Input: part model. Units: mm. Frame: model coordinates. Face numbers are marked on the shaded views. A direction names the side the tool comes from. Give positions to 0.01 mm unless a question says otherwise; leave off trailing zeros. Order: outer loops, then holes, each group sorted by start corner. A loop starts at its lowest first (then second) coordinate and runs counter-clockwise, first axis right, second up.
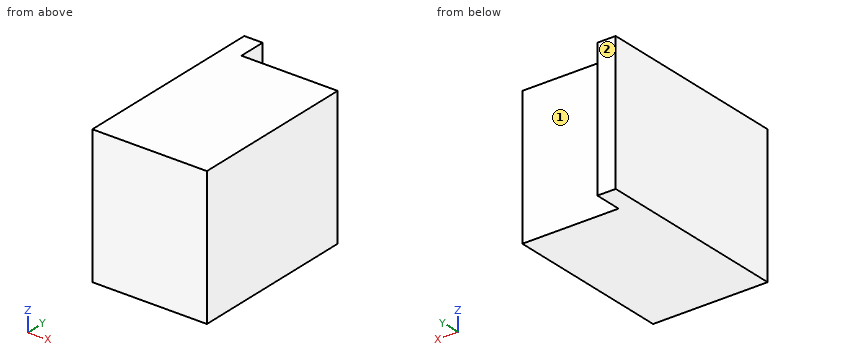
Autodesk Inventor part; units mm, degrees
ref_plane "YZ Plane" through (0, 0, 0) normal (1, 0, 0) x (0, 1, 0)
ref_plane "XZ Plane" through (0, 0, 0) normal (0, 1, 0) x (-1, 0, 0)
ref_plane "XY Plane" through (0, 0, 0) normal (0, 0, 1) x (1, 0, 0)
sketch "Sketch1" plane through (0, 0, 0) normal (0, 1, 0) x (-1, 0, 0)
  line L0 (0, 0) -> (-635, 0)
  line L1 (-635, 0) -> (-635, -762)
  line L2 (-635, -762) -> (0, -762)
  line L3 (0, -762) -> (0, 0)
  dimension "d4" = 762
  dimension "d5" = 635
extrude "Extrusion1" add sketch "Sketch1" along normal blind 939.8
sketch "Sketch2" plane through (0, 939.8, 0) normal (0, 1, 0) x (1, 0, 0)
  line L0 (0, 762) -> (0, 0)
  line L1 (0, 0) -> (635, 0)
  line L2 (0, 762) -> (101.6, 762)
  line L3 (101.6, 762) -> (101.6, 0)
  line L4 (101.6, 0) -> (0, 0)
  line L5 (0, 0) -> (0, 762)
  dimension "d6" = 101.6
extrude "Extrusion2" add sketch "Sketch2" along normal blind 152.4
properties part number "Stove" material "Stainless Steel"
1) Cut plane C-C (y = 972). Return the cut outline in (x, z), then the cut area to 3 significant figures.
2) Reachability of the marked faces 1 and 2 from +Z, -Z, +X, -X, +Y, -Y: full face, straight path, thin tool, end or side. Return the list, or none.
3) First-contact query: P1, Ø4, axis at x = 307, z = -242.5, coming from the +Y side. Flat tip, straight axial feed; report the tip coordinate or a pass-through.
4) Line query: probe 1 along Y at (x, z) = (234, -639); probe 2 along X at (y, z) = (1012, -572.5). Output: solid intervals per line, ascending.
5) Cut plane A-A (z = -182.5). Return the cut outline in (x, y).
6) Cut plane B-B (x = 522). Return the cut outline in (y, z), then the cut area to 3 significant figures.
Geometry says:
1. outline: (0, -762) - (101.6, -762) - (101.6, 0) - (0, 0) - close
1. area: 77,400 mm2
2. face 1: +Z, -Z, +X, +Y
2. face 2: +Z, -Z, +X, -X, +Y
3. P1: stops at y = 939.8
4. probe 1: y = 0 to 939.8
4. probe 2: x = 0 to 101.6
5. outline: (0, 0) - (635, 0) - (635, 939.8) - (101.6, 939.8) - (101.6, 1092.2) - (0, 1092.2) - close
6. outline: (0, -762) - (939.8, -762) - (939.8, 0) - (0, 0) - close
6. area: 716,000 mm2
